Part print with two shaded views. Sizes in mm from the minimum x, y, z corner. A direction names the side the tool comes from. Give positions to 0.01 mm unless a question says otherwise; leave off trailing zeros. Write each loop counter-clockwise with the first axis right and the second up, starting at its lowest first coordinate (ties: lowest second). Pieces come first, ordered by that corner, then holes. Notation, with made-up numbers: (77.25, -27) -> (130.25, -27) arc R23 cw to (130.25, 3) -> close; hole circle Ø6 at (-13, 68.25). An arc over 180 degrees is marked (long way). Answer as a JSON object with one key per item and string values.
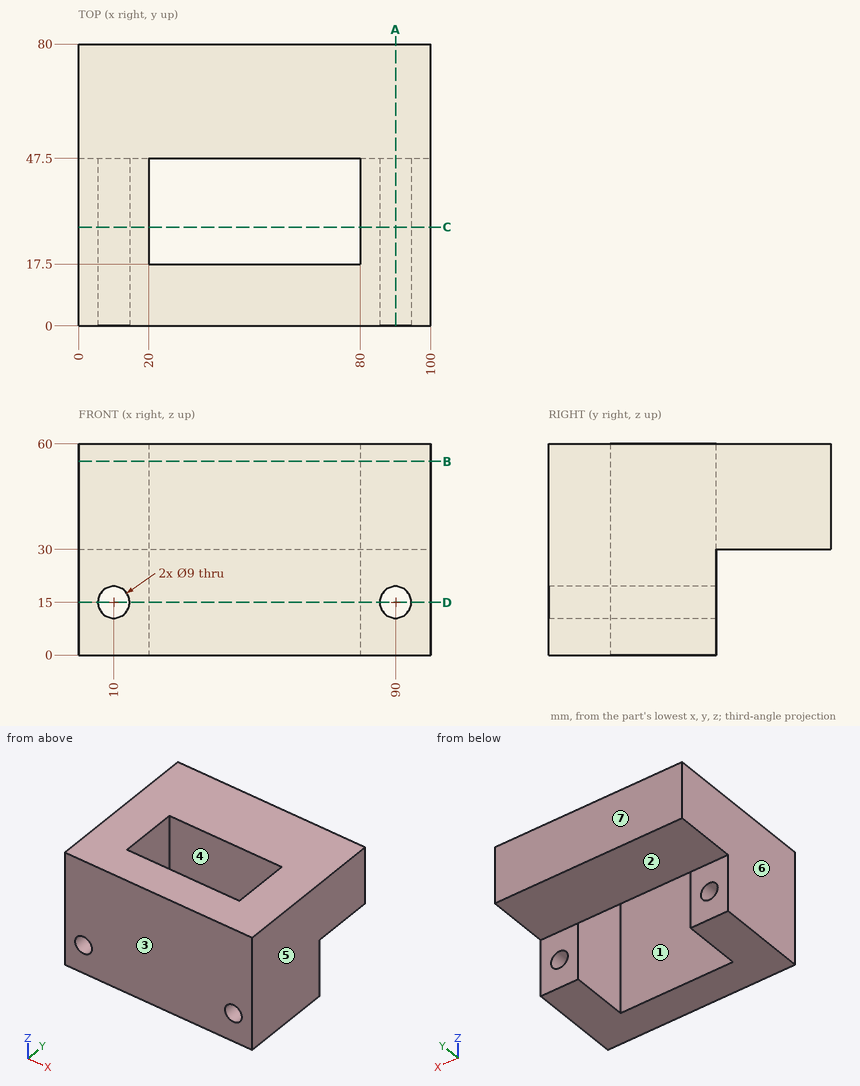
1) Slice it at A-A (x = 90). List the corners of the cut face in (y, z), then the cut area to 3 significant figures.
Model answer:
{"outline": "(0, 0) -> (47.5, 0) -> (47.5, 10.5) -> (0, 10.5) -> close; (0, 19.5) -> (47.5, 19.5) -> (47.5, 30) -> (80, 30) -> (80, 60) -> (0, 60) -> close", "area": "3,400 mm2"}
2) Slice it at B-B (z = 55). List the corners of the cut face in (x, y).
Model answer:
{"outline": "(0, 0) -> (100, 0) -> (100, 80) -> (0, 80) -> close; hole (20, 17.5) -> (80, 17.5) -> (80, 47.5) -> (20, 47.5) -> close"}
3) Pin check, flat tips, straight feed: pin 1 (6 mm diameter, centred on x = 94.5, z = 21, fed in from +Y); pin 2 (12 mm diameter, centred on x = 75, y = 61, fed in from -Z). Stop position of each tip, or through.
Model answer:
{"pin 1": "stops at y = 47.5", "pin 2": "stops at z = 30"}
4) Slice it at D-D (z = 15). List the corners of the cut face in (x, y), then the cut area to 4 significant figures.
Model answer:
{"outline": "(0, 0) -> (5.5, 0) -> (5.5, 47.5) -> (0, 47.5) -> close; (14.5, 0) -> (85.5, 0) -> (85.5, 47.5) -> (80, 47.5) -> (80, 17.5) -> (20, 17.5) -> (20, 47.5) -> (14.5, 47.5) -> close; (94.5, 0) -> (100, 0) -> (100, 47.5) -> (94.5, 47.5) -> close", "area": "2,095 mm2"}
5) Wall check: probe 1 along X at (y, z) = (20.5, 15); probe 2 along X at (y, z) = (11, 15); probe 3 along X at (y, z) = (46.5, 52). Give the ranges that are in metal, low to high.
Model answer:
{"probe 1": "x = 0 to 5.5, 14.5 to 20, 80 to 85.5, 94.5 to 100", "probe 2": "x = 0 to 5.5, 14.5 to 85.5, 94.5 to 100", "probe 3": "x = 0 to 20, 80 to 100"}
6) Slice it at C-C (y = 28). List the corners of the cut face in (x, z).
Model answer:
{"outline": "(0, 0) -> (20, 0) -> (20, 60) -> (0, 60) -> close; (80, 0) -> (100, 0) -> (100, 60) -> (80, 60) -> close; hole circle Ø9 at (10, 15); hole circle Ø9 at (90, 15)"}
7) Mould opens along X. For the marked faces 4, 5, 6 and 7 say: released by +X, released by -X, zero draft, split by the parting line, or undercut.
Model answer:
{"face 4": "undercut", "face 5": "released by +X", "face 6": "released by -X", "face 7": "zero draft"}
8) 3-axis set-ups, long thin cutter, end or side, ignore diameter. For the marked faces 1, 2 and 3: which of +Z, -Z, +X, -X, +Y, -Y reach the whole face in a straight line?
Model answer:
{"face 1": "+Z, -Z", "face 2": "-Z, +X, -X, +Y", "face 3": "+Z, -Z, +X, -X, -Y"}
